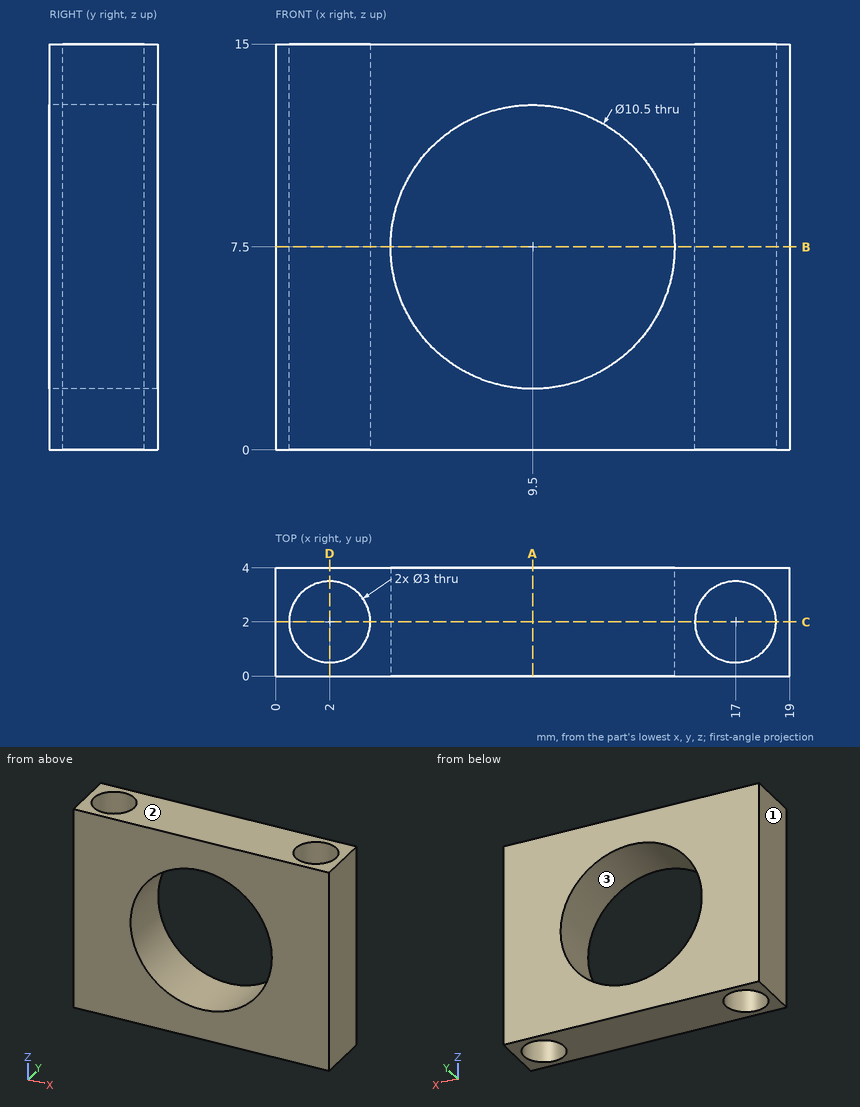
Geometry: see drawing. Coordinates: mm, zero at the bounding-box minimum. Coordinates: 2 decimals unless noted, no trailing zeros. Write each loop counter-clockwise with the first axis right and the second up, starting at its lowest first coordinate (ties: lowest second). Pieces come first, ordered by that corner, then holes. Notation, with made-up numbers: (29, 24.5) - (38, 24.5) arc R18 cw to (38, 56.5) - close; hole circle Ø7 at (55.25, 20). An arc over 180 degrees is marked (long way). Put each result on its own line as item: value. Start each with the question number.
1) Cut plane B-B (z = 7.5). Return the cut outline in (x, y), plus the area to 3 significant figures.
2) Cut plane C-C (y = 2). Return the cut outline in (x, z).
3) Ray query, L1, parallel to Z at x = 9.5, y = 1.1; L2, parallel to Y at x = 17, z = 11.5; L3, parallel to X at y = 2.35, z = 9.25. Return the intervals inside material, ascending.
4) Cut plane A-A (x = 9.5). Return the cut outline in (y, z), plus the area to 3 significant figures.
5) Cut plane D-D (x = 2). Return the cut outline in (y, z).
6) Mould query, pull axis X, two halves, no side actions, for the marked faces 1, 2 and 3. Classes: pulls with the +X half, pulls with the -X half, needs draft (parallel to the pull), parting line crosses it, or undercut.
Resolved:
1. outline: (0, 0) - (4.25, 0) - (4.25, 4) - (0, 4) - close; (14.75, 0) - (19, 0) - (19, 4) - (14.75, 4) - close; hole circle Ø3 at (2, 2); hole circle Ø3 at (17, 2)
1. area: 19.9 mm2
2. outline: (0, 0) - (0.5, 0) - (0.5, 15) - (0, 15) - close; (3.5, 0) - (15.5, 0) - (15.5, 15) - (3.5, 15) - close; (18.5, 0) - (19, 0) - (19, 15) - (18.5, 15) - close; hole circle Ø10.5 at (9.5, 7.5)
3. L1: z = 0 to 2.25, 12.75 to 15
3. L2: y = 0 to 0.5, 3.5 to 4
3. L3: x = 0 to 0.54, 3.46 to 4.55, 14.45 to 15.54, 18.46 to 19
4. outline: (0, 0) - (4, 0) - (4, 2.25) - (0, 2.25) - close; (0, 12.75) - (4, 12.75) - (4, 15) - (0, 15) - close
4. area: 18.0 mm2
5. outline: (0, 0) - (0.5, 0) - (0.5, 15) - (0, 15) - close; (3.5, 0) - (4, 0) - (4, 15) - (3.5, 15) - close
6. face 1: pulls with the -X half
6. face 2: needs draft
6. face 3: undercut
